from build123d import *

# Parameters (mm, degrees)
SKETCH_1_R                   = 60
EXTRUDE_1_DEPTH              = 7.5
SKETCH_2_R                   = 27.5
CUT_EXTRUDE_1_DEPTH          = 16
SKETCH_3_R                   = 45
SKETCH_3_R_2                 = 41
CUT_EXTRUDE_2_DEPTH          = 0.5
HOLE_WIZARD_M5_1_D           = 5.5
HOLE_WIZARD_M5_1_CBORE_D     = 9.5
HOLE_WIZARD_M5_1_CBORE_DEPTH = 5.4
M5X0_8_1_D                   = 4.2
PATTERN_CIRCULAR_1_COUNT     = 8


with BuildPart() as part:
    # 草圖1 → 填料-伸長1 (new body, symmetric)
    with BuildSketch(Plane.XY):
        Circle(SKETCH_1_R)
    extrude(amount=EXTRUDE_1_DEPTH, both=True)

    # 草圖2 → 除料-伸長1 (cut, through all)
    with BuildSketch(Plane.XY.offset(7.5)):
        Circle(SKETCH_2_R)
    extrude(amount=-CUT_EXTRUDE_1_DEPTH, mode=Mode.SUBTRACT)

    # 草圖3 → 除料-伸長2 (cut)
    with BuildSketch(Plane.XY.offset(7.5)):
        Circle(SKETCH_3_R)
        Circle(SKETCH_3_R_2, mode=Mode.SUBTRACT)
    cut_extrude_2 = extrude(amount=-CUT_EXTRUDE_2_DEPTH, mode=Mode.SUBTRACT)

    # 鏡射1: 除料-伸長2 across plane
    add(cut_extrude_2.mirror(Plane.XY), mode=Mode.SUBTRACT)

    # M5 凹頭蓋螺釘的柱孔1 (through all)
    with Locations(Plane.XY.offset(7.5)):
        with Locations((0, 52.5)):
            hole_wizard_m5_1 = CounterBoreHole(HOLE_WIZARD_M5_1_D / 2, HOLE_WIZARD_M5_1_CBORE_D / 2, HOLE_WIZARD_M5_1_CBORE_DEPTH)

    # M5x0.8 螺紋孔1 (through all)
    with Locations(Plane.XY.offset(7.5)):
        with Locations((0, 32.5)):
            m5x0_8_1 = Hole(M5X0_8_1_D / 2)

    # 環狀複製排列1: M5 凹頭蓋螺釘的柱孔1, M5x0.8 螺紋孔1 ×8 about axis
    pattern_circular_1_axis = Axis((0, 0, 0), (0, 0, 1))
    for i in range(1, PATTERN_CIRCULAR_1_COUNT):
        add(hole_wizard_m5_1.rotate(pattern_circular_1_axis, i * 360 / PATTERN_CIRCULAR_1_COUNT), mode=Mode.SUBTRACT)
        add(m5x0_8_1.rotate(pattern_circular_1_axis, i * 360 / PATTERN_CIRCULAR_1_COUNT), mode=Mode.SUBTRACT)


solid = part.part
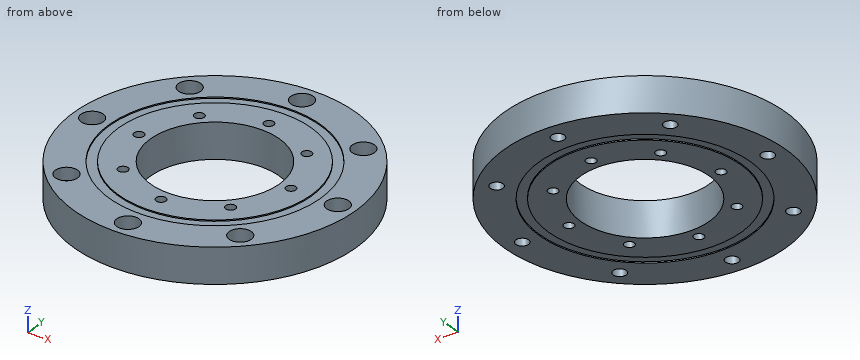
Could you check a few things on this model? Use its own coordinates, in mm. Give positions to 0.01 mm unless a question says otherwise; leave off trailing zeros. Order: outer loops, then holes, each group sorted by start corner. A loop starts at its lowest first (then second) coordinate and runs counter-clockwise, first axis right, second up. Notation, with made-up numbers: (-5.5, 70.5) -> (5.5, 70.5) arc R19 cw to (5.5, 106.5) -> close; hole circle Ø7 at (-22.75, 59.5). An arc over 180 degrees is marked (long way). Answer in a Markdown table with one row per item. Add a question column.
Item 1: Imagine slicing it at A-A (x = -52.5). List the corners of the cut face in (y, z) for me.
Item 2: I'm going to push flat-ended pins straight in: P1, Ø8, axis at x = -25, z = 4, coming from the +Y side (3 decimals); P2, Ø7, axis at x = -37.12, y = 37.12, coming from the +Z side; P3, Ø6, axis at y = -9, z = -5, coming from the -X side. Where does each tip first touch, or does it pass through?
Item 3: Imagine slicing it at D-D (y = 18). List the corners of the cut face in (x, z) for me, and give its area (3 significant figures).
Item 4: Please list where these lines run through material, in increasing order: probe 1 along Y at (x, z) = (22.5, -4.5); probe 2 along X at (y, z) = (35, 1); probe 3 along X at (y, z) = (24.5, 4.5).
Item 5: Imagine slicing it at B-B (y = -8.5). List the corners of the cut face in (x, z) for me.
Item 6: Imagine slicing it at C-C (z = 5). Count the separate pieces of the cut face and the enclosed holes in it, and give its area (3 significant figures).
Result:
| question | item | result |
|---|---|---|
| 1 | outline | (-29.05, -7.5) -> (-2.75, -7.5) -> (-2.75, 2.1) -> (-4.75, 2.1) -> (-4.75, 7.5) -> (-29.05, 7.5) -> close; (2.75, -7.5) -> (29.05, -7.5) -> (29.05, 7.5) -> (4.75, 7.5) -> (4.75, 2.1) -> (2.75, 2.1) -> close |
| 2 | P1 | y = 56.205 |
| 2 | P2 | z = 2.1 |
| 2 | P3 | x = -59.7 |
| 3 | outline | (-57.24, -7.5) -> (-41.24, -7.5) -> (-41.24, -7) -> (-36.84, -7) -> (-36.84, -7.5) -> (-20.79, -7.5) -> (-20.79, 7.5) -> (-36.84, 7.5) -> (-36.84, 7) -> (-41.24, 7) -> (-41.24, 7.5) -> (-57.24, 7.5) -> close; (20.79, -7.5) -> (36.84, -7.5) -> (36.84, -7) -> (41.24, -7) -> (41.24, -7.5) -> (57.24, -7.5) -> (57.24, 7.5) -> (41.24, 7.5) -> (41.24, 7) -> (36.84, 7) -> (36.84, 7.5) -> (20.79, 7.5) -> close |
| 3 | area | 1,080 mm2 |
| 4 | probe 1 | -55.62 to -25.03, -20.94 to -15.81, 15.81 to 20.94, 25.03 to 55.62 |
| 4 | probe 2 | -48.73 to -38.87, -35.38 to 35.38, 38.87 to 48.73 |
| 4 | probe 3 | -54.77 to -24.43, -21.53 to -12.49, 12.49 to 21.53, 24.43 to 54.77 |
| 5 | outline | (-59.39, -7.5) -> (-44.19, -7.5) -> (-44.19, -7) -> (-40.11, -7) -> (-40.11, -7.5) -> (-26.15, -7.5) -> (-26.15, 7.5) -> (-40.11, 7.5) -> (-40.11, 7) -> (-44.19, 7) -> (-44.19, 7.5) -> (-59.39, 7.5) -> close; (26.15, -7.5) -> (40.11, -7.5) -> (40.11, -7) -> (44.19, -7) -> (44.19, -7.5) -> (59.39, -7.5) -> (59.39, 7.5) -> (44.19, 7.5) -> (44.19, 7) -> (40.11, 7) -> (40.11, 7.5) -> (26.15, 7.5) -> close |
| 6 | separate pieces | 1 |
| 6 | enclosed holes | 17 |
| 6 | area | 8,260 mm2 |
